from build123d import *

# Parameters (mm, degrees)
CROQUIS1_R              = 1.59
CROQUIS1_R_2            = 1.5875
CROQUIS1_R_3            = 4
SALIENTE_EXTRUIR1_DEPTH = 5


with BuildPart() as part:
    # Croquis1 → Saliente-Extruir1 (new body)
    with BuildSketch(Plane.XY):
        with BuildLine():
            ThreePointArc((1.193677036, 26.351337281), (0.615813463, 26.577686227), (0, 26.654718258))
            ThreePointArc((0, 26.654718258), (-0.615813463, 26.577686227), (-1.193677036, 26.351337281))
            Line((-1.193677036, 26.351337281), (-2.643396871, 25.563536913))
            ThreePointArc((-2.643396871, 25.563536913), (-3.37085174, 24.966684186), (-3.826144074, 24.143196083))
            Line((-3.826144074, 24.143196083), (-9.459133033, 6.898899359))
            ThreePointArc((-9.459133033, 6.898899359), (-9.492428214, 4.521789334), (-8.170864273, 2.54562401))
            ThreePointArc((-8.170864273, 2.54562401), (-7.560847643, 1.822599507), (-7.263149059, 0.924679537))
            ThreePointArc((-7.263149059, 0.924679537), (-7.323699332, -0.668363985), (-7.905472696, -2.152612532))
            ThreePointArc((-7.905472696, -2.152612532), (-8.1122929, -2.44647205), (-8.359106022, -2.707644973))
            ThreePointArc((-8.359106022, -2.707644973), (-9.655003955, -5.778505112), (-8.174803271, -8.764897481))
            Line((-8.174803271, -8.764897481), (-6.609038667, -11.365635857))
            ThreePointArc((-6.609038667, -11.365635857), (-5.007106824, -15.087530614), (-4.459817284, -19.102398031))
            Line((-4.459817284, -19.102398031), (-4.459817284, -20))
            Line((-4.459817284, -20), (-5.626230736, -80))
            Line((-5.626230736, -80), (-5.626230736, -82.958659211))
            add(Edge.make_bspline(
                [(-5.626230736, -82.958659211), (-3.957996586, -86.469029482), (-1.373693138, -88.776535361), (1.33959564, -91.266262586)],
                knots=[0, 0, 0, 0, 0.775055833, 0.775055833, 0.775055833, 0.775055833], degree=3))
            Line((1.33959564, -91.266262586), (7.160508284, -96.56338139))
            Line((7.160508284, -96.56338139), (11.535313635, -91.755983118))
            Line((11.535313635, -91.755983118), (9.058275941, -89.496367102))
            ThreePointArc((9.058275941, -89.496367102), (6.055620379, -85.213180579), (5.626230736, -80))
            Line((5.626230736, -80), (4.459817284, -20))
            Line((4.459817284, -20), (4.459817284, -19.102398031))
            ThreePointArc((4.459817284, -19.102398031), (5.007106824, -15.087530614), (6.609038667, -11.365635857))
            Line((6.609038667, -11.365635857), (8.174803271, -8.764897481))
            ThreePointArc((8.174803271, -8.764897481), (9.655003955, -5.778505112), (8.359106022, -2.707644973))
            ThreePointArc((8.359106022, -2.707644973), (8.1122929, -2.44647205), (7.905472696, -2.152612532))
            ThreePointArc((7.905472696, -2.152612532), (7.323699332, -0.668363985), (7.263149059, 0.924679537))
            ThreePointArc((7.263149059, 0.924679537), (7.560847643, 1.822599507), (8.170864273, 2.54562401))
            ThreePointArc((8.170864273, 2.54562401), (9.492428214, 4.521789334), (9.459133033, 6.898899359))
            Line((9.459133033, 6.898899359), (3.826144074, 24.143196083))
            ThreePointArc((3.826144074, 24.143196083), (3.37085174, 24.966684186), (2.643396871, 25.563536913))
            Line((2.643396871, 25.563536913), (1.193677036, 26.351337281))
        make_face()
        with Locations((-1.416184287, -81.918657321)):
            Circle(CROQUIS1_R, mode=Mode.SUBTRACT)
        with Locations((0.39268377, -71.387686118)):
            Circle(CROQUIS1_R_2, mode=Mode.SUBTRACT)
        with BuildLine():
            ThreePointArc((-5.091168825, -7.283199846), (-7.283199846, -7.283199846), (-7.283199846, -5.091168825))
            Line((-7.283199846, -5.091168825), (-6.222539674, -4.030508653))
            ThreePointArc((-6.222539674, -4.030508653), (-4.030508653, -4.030508653), (-4.030508653, -6.222539674))
            Line((-4.030508653, -6.222539674), (-5.091168825, -7.283199846))
        make_face(mode=Mode.SUBTRACT)
        with BuildLine():
            ThreePointArc((-7.283199846, 5.091168825), (-7.283199846, 7.283199846), (-5.091168825, 7.283199846))
            Line((-5.091168825, 7.283199846), (-4.030508653, 6.222539674))
            ThreePointArc((-4.030508653, 6.222539674), (-4.030508653, 4.030508653), (-6.222539674, 4.030508653))
            Line((-6.222539674, 4.030508653), (-7.283199846, 5.091168825))
        make_face(mode=Mode.SUBTRACT)
        Circle(CROQUIS1_R_3, mode=Mode.SUBTRACT)
        with BuildLine():
            Line((-3.690213899, 12.181248638), (-2.502144822, 19.079689902))
            ThreePointArc((-2.502144822, 19.079689902), (-1.635896096, 20.590481825), (0, 21.187744795))
            ThreePointArc((0, 21.187744795), (1.635896096, 20.590481825), (2.502144822, 19.079689902))
            Line((2.502144822, 19.079689902), (3.707704632, 12.079689902))
            add(Edge.make_bspline(
                [(3.707704632, 12.079689902), (-0.039943984, 7.807746472), (-3.690213899, 12.181248638)],
                knots=[0.502108549, 0.502108549, 0.502108549, 1.502108549, 1.502108549, 1.502108549], degree=2))
        make_face(mode=Mode.SUBTRACT)
        with BuildLine():
            ThreePointArc((7.283199846, -5.091168825), (7.283199846, -7.283199846), (5.091168825, -7.283199846))
            Line((5.091168825, -7.283199846), (4.030508653, -6.222539674))
            ThreePointArc((4.030508653, -6.222539674), (4.030508653, -4.030508653), (6.222539674, -4.030508653))
            Line((6.222539674, -4.030508653), (7.283199846, -5.091168825))
        make_face(mode=Mode.SUBTRACT)
        with BuildLine():
            Line((4.560838717, 6.752869739), (5.091168825, 7.283199846))
            ThreePointArc((5.091168825, 7.283199846), (7.283199846, 7.283199846), (7.283199846, 5.091168825))
            Line((7.283199846, 5.091168825), (6.752869872, 4.56083885))
            ThreePointArc((6.752869872, 4.56083885), (4.560838805, 4.560838672), (4.560838717, 6.752869739))
        make_face(mode=Mode.SUBTRACT)
    extrude(amount=SALIENTE_EXTRUIR1_DEPTH)


solid = part.part
Can you work these out from the model? Positions are in its coordinate system, mm. A direction names the side the tool comes from. Round coordinates to 2 decimals unless told otherwise and drop trailing zeros. Write each loop counter-clockwise with the first axis right and the second up, starting at its lowest first coordinate (ties: lowest second). Pieces come first, ordered by that corner, then holes. Notation, with made-up numbers: M 33,75.25 L 81,75.25 A6 ccw 81,80.25 Z; hole C 58,22 d1. An arc over 180 degrees is marked long. Use a Markdown table: item, result.
Item 1: I want a section at A-A (z = 2.85). State how many separate pieces and enclosed holes the cut face has, and give its area (3 significant figures).
Found:
| item | result |
|---|---|
| separate pieces | 1 |
| enclosed holes | 8 |
| area | 1,220 mm2 |
Item 2: I want a section at C-C (y = -43). List the corners of the cut face in (x, z) for me.
Found:
| item | result |
|---|---|
| outline | M -4.91,0 L 4.91,0 L 4.91,5 L -4.91,5 Z |
Item 3: I want a section at B-B (y = -65.5). List the corners of the cut face in (x, z) for me, and give its area (3 significant figures).
Found:
| item | result |
|---|---|
| outline | M -5.34,0 L 5.34,0 L 5.34,5 L -5.34,5 Z |
| area | 53.4 mm2 |
Item 4: For pin 1 Ø10 at (x, y) = (8.5, 3.5) entering from -Z; pin 2 Ø2 at (x, z) = (0.5, 3) entering from -Y; pin 3 Ø1.9 at (x, y) = (-1.42, -81.92) entering from -Z; pin 4 Ø1.5 at (y, z) = (-82, 3) entering from -X, each with a flat end and sliding along its axis, tell me the tip position at first contact or that it passes through.
Found:
| item | result |
|---|---|
| pin 1 | stops at z = 0 |
| pin 2 | stops at y = -91.41 |
| pin 3 | passes through |
| pin 4 | stops at x = -5.63 |
Item 5: We'd pull the mould along Y, two halves only. Please class faces 1 (the face through (4.01, -4.05, 2.46)), 2 (the face through (9.32, -94.19, 2.46)), 3 (the face through (-5.626, -81, 2)): released by +Y, released by -Y, zero draft, split by the parting line, or undercut.
Found:
| item | result |
|---|---|
| face 1 | undercut |
| face 2 | released by -Y |
| face 3 | zero draft |
Item 6: If I drill on line 1 along Y through (x, z) = (1.25, 2.65); line 2 along X through (y, z) = (4.5, 1.15); line 3 along X through (y, z) = (13.5, 3.8), over which ranges is the centre line in solid material (lowest first)? Write a range as [from, to].
Found:
| item | result |
|---|---|
| line 1 | y = [-91.18, -72.72], [-70.05, -3.8], [3.8, 10.2], [20.86, 26.32] |
| line 2 | x = [-9.49, -6.69], [-3.71, 4.63], [6.69, 9.49] |
| line 3 | x = [-7.3, -3.46], [3.46, 7.3] |
Item 7: Which directions (+Z, -Z, +X, -X, +Y, -Y) give clear straight access to the entire face, cutting with the end or side of a thin tool? Please do faces 4 (the face through (-3.1, 15.6, 2.5)), 5 (the face through (1, -34, 5)), 6 (the face through (-5.022, -15.033, 2.465)), 7 (the face through (4.992, -15.142, 2.465)), 8 (the face through (4.21, -93.88, 2.46)).
Found:
| item | result |
|---|---|
| face 4 | +Z, -Z |
| face 5 | +Z, +X, -X, +Y, -Y |
| face 6 | +Z, -Z, -X |
| face 7 | +Z, -Z, +X |
| face 8 | +Z, -Z, -X, -Y |
